Geometry: final body of the model. Coordinates: model frame, mm. A direction names the side the tool comes from. Give positions to 0.01 mm unless a question says otherwise; leave off trailing zeros. Loops run counter-clockwise (first coordinate to the right, second up) from the corner with the lowest first, then second, coordinate; pieces in that order, holes last. Notation, with made-up numbers: (24.5, -24.75) -> (49.5, -24.75) arc R32 ccw to (49.5, 11.25) -> close; hole circle Ø11 at (0, 49.5). An arc over 180 degrees is marked (long way). Answer in a Markdown table with one row per item. Add a question column.
from build123d import *

# Parameters (mm, degrees)
BOSS_EXTRUDE1_DEPTH = 20
SKETCH2_R           = 3
CUT_EXTRUDE1_DEPTH  = 3
BOSS_EXTRUDE2_START = 7
SKETCH3_W           = 17
SKETCH3_H           = 17
SKETCH3_R           = 3
BOSS_EXTRUDE2_DEPTH = 7
SKETCH4_R           = 6.5
CUT_EXTRUDE2_DEPTH  = 5
FILLET1_R           = 3


with BuildPart() as part:
    # Sketch1 → Boss-Extrude1 (new body)
    with BuildSketch(Plane(origin=(0, 0, 0), x_dir=(0, 0, -1), z_dir=(1, 0, 0))):
        Polygon((2.785388085, -22.866116346), (4.285388085, -22.866116346), (4.285388085, -20.866116346), (0.285388085, -20.866116346), (0.285388085, -43.366116346), (4.285388085, -43.366116346), (4.285388085, -41.366116346), (2.785388085, -41.366116346), align=None)
    extrude(amount=BOSS_EXTRUDE1_DEPTH)

    # Sketch2 → Cut-Extrude1 (cut)
    with BuildSketch(Plane.XY.offset(-0.285388085)):
        with Locations((9, -32.116116346)):
            Circle(SKETCH2_R)
    extrude(amount=-CUT_EXTRUDE1_DEPTH, mode=Mode.SUBTRACT)

    # Sketch3 → Boss-Extrude2 (add)
    with BuildSketch(Plane.XY.offset(-0.285388085).offset(BOSS_EXTRUDE2_START)):
        with Locations((9, -32.116116346)):
            Rectangle(SKETCH3_W, SKETCH3_H)
        with Locations((9, -32.116116346)):
            Circle(SKETCH3_R, mode=Mode.SUBTRACT)
    extrude(amount=-BOSS_EXTRUDE2_DEPTH)

    # Sketch4 → Cut-Extrude2 (cut)
    with BuildSketch(Plane.XY.offset(6.714611915)):
        with Locations((9, -32.116116346)):
            Circle(SKETCH4_R)
    extrude(amount=-CUT_EXTRUDE2_DEPTH, mode=Mode.SUBTRACT)

    # Fillet1
    fillet1_edges = [part.edges().sort_by_distance(p)[0] for p in [
        (0.5, -23.616116346, 3.214611915),
        (0.5, -40.616116346, 3.214611915),
        (17.5, -40.616116346, 3.214611915),
        (17.5, -23.616116346, 3.214611915),
    ]]
    fillet(fillet1_edges, radius=FILLET1_R)


solid = part.part
(1) Cut plane D-D on x = 12.75. Return the cut outline in (y, z).
(2) Pin query (flat end, axial travel): pin 1 Ø3 at (x, y) = (6.5, -26.5) entering from -Z; pin 2 Ø2 at (y, z) = (-29.5, 5) entering from +X; pin 3 Ø1 at (y, z) = (-28.5, -2) entering from -X; pin 4 Ø2 at (x, z) = (6.5, 2) entering from +Y. Return the tip coordinate at first contact, or that it passes through.
(3) Material intervals for line 1 along Y through (x, z) = (9, 0); line 2 along Y through (x, z) = (9, 5.75); line 3 along Z through (x, y) = (6, -22.25), sorted ascending. Write a range as from..to.
(4) Reachability of faces 1 (the flat face through (10, -22.866, -4)), 2 (the flat face through (9, -40.616, 3)), 3 (the cylindrical face through (1.355, -39.714, 3.166)) from +Z, -Z, +X, -X, +Y, -Y: full face, straight path, thin tool, end or side. Return the list, or none.
(5) Cut plane C-C on z = 3.75. Return the cut outline in (x, y), then the cut area to 3 significant figures.
(6) Cut plane B-B on y = -34. Return the cut outline in (x, z).
(7) Cut plane A-A on x = 9. Return the cut outline in (y, z), then the cut area to 4 significant figures.
(8) Draft query along Y for faces 4 (the cylindrical face through (7.59, -38.46, 4.25)), 5 (the flat face through (17.5, -32, 3)), 6 (the cylindrical face through (16.598, -24.472, 3.166)). Return one class per face: +Y half, -Y half, draft (parallel to the pull), parting line (faces both ways), or undercut.
Answer list:
| question | item | result |
|---|---|---|
| 1 | outline | (-43.37, -4.29) -> (-41.37, -4.29) -> (-41.37, -2.79) -> (-22.87, -2.79) -> (-22.87, -4.29) -> (-20.87, -4.29) -> (-20.87, -0.29) -> (-23.62, -0.29) -> (-23.62, 6.71) -> (-26.81, 6.71) -> (-26.81, 1.71) -> (-37.43, 1.71) -> (-37.43, 6.71) -> (-40.62, 6.71) -> (-40.62, -0.29) -> (-43.37, -0.29) -> close |
| 2 | pin 1 | stops at z = -2.79 |
| 2 | pin 2 | stops at x = 17.5 |
| 2 | pin 3 | stops at x = 0 |
| 2 | pin 4 | stops at y = -23.62 |
| 3 | line 1 | y = -40.62..-35.12, -29.12..-23.62 |
| 3 | line 2 | y = -40.62..-38.62, -25.62..-23.62 |
| 3 | line 3 | z = -4.29..-0.29 |
| 4 | face 1 | -Z, +X, -X |
| 4 | face 2 | +Z, +X, -X, -Y |
| 4 | face 3 | +Z, -X, -Y |
| 5 | outline | (0.5, -37.62) arc R3 ccw to (3.5, -40.62) -> (14.5, -40.62) arc R3 ccw to (17.5, -37.62) -> (17.5, -26.62) arc R3 ccw to (14.5, -23.62) -> (3.5, -23.62) arc R3 ccw to (0.5, -26.62) -> close; hole circle Ø13 at (9, -32.12) |
| 5 | area | 149 mm² |
| 6 | outline | (0, -2.79) -> (6.67, -2.79) -> (6.67, 1.71) -> (2.78, 1.71) -> (2.78, 6.71) -> (0.5, 6.71) -> (0.5, -0.29) -> (0, -0.29) -> close; (11.33, -2.79) -> (20, -2.79) -> (20, -0.29) -> (17.5, -0.29) -> (17.5, 6.71) -> (15.22, 6.71) -> (15.22, 1.71) -> (11.33, 1.71) -> close |
| 7 | outline | (-43.37, -4.29) -> (-41.37, -4.29) -> (-41.37, -2.79) -> (-35.12, -2.79) -> (-35.12, 1.71) -> (-38.62, 1.71) -> (-38.62, 6.71) -> (-40.62, 6.71) -> (-40.62, -0.29) -> (-43.37, -0.29) -> close; (-29.12, -2.79) -> (-22.87, -2.79) -> (-22.87, -4.29) -> (-20.87, -4.29) -> (-20.87, -0.29) -> (-23.62, -0.29) -> (-23.62, 6.71) -> (-25.62, 6.71) -> (-25.62, 1.71) -> (-29.12, 1.71) -> close |
| 7 | area | 89.25 mm² |
| 8 | face 4 | undercut |
| 8 | face 5 | draft |
| 8 | face 6 | +Y half |
